from build123d import *

# Parameters (mm, degrees)
F0_R        = 4.945
F0_R_2      = 3.445
F1_DEPTH    = 4
F0_R_3      = 6.945
F1_FACE_R   = 4.945
F1_FACE_R_2 = 3.445
F2_DEPTH    = 1
F3_SIZE     = 0.99999
F4_SIZE2    = 1
F4_SIZE     = 1


# Not quite as in the source:
# - a fillet or chamfer is up to 0.001 mm smaller than in the source, because OpenCascade refuses the exact size


with BuildPart() as f1:
    # F0 (on Top) → F1 (new body)
    with BuildSketch(Plane.XY):
        Circle(F0_R)
        Circle(F0_R_2, mode=Mode.SUBTRACT)
    extrude(amount=-F1_DEPTH)

    # F0 (on Top) + F1_face (on face) → F2 (join)
    with BuildSketch(Plane.XY):
        Circle(F0_R_3)
        Circle(F0_R, mode=Mode.SUBTRACT)
        Circle(F0_R_2)
    with BuildSketch(Plane.XY):
        Circle(F1_FACE_R)
        Circle(F1_FACE_R_2, mode=Mode.SUBTRACT)
    extrude(amount=F2_DEPTH)

    # F3 (size 1 in the source; OpenCascade refuses exactly that, so slightly less here)
    f3_edges = [f1.edges().sort_by_distance(p)[0] for p in [
        (-6.945, 0, 1),
    ]]
    chamfer(f3_edges, length=F3_SIZE)

    # F4
    f4_edges = [f1.edges().sort_by_distance(p)[0] for p in [
        (-4.945, 0, -4),
    ]]
    chamfer(f4_edges, length=F4_SIZE, length2=F4_SIZE2)


solid = f1.part
Input: part model. Units: mm. Frame: model coordinates. A direction names the side the tool comes from. Coordinates: 2 decimals unless noted, no trailing zeros. Loops run counter-clockwise (first coordinate to the right, second up) from the corner with the lowest first, then second, coordinate; pieces in that order, holes last.
Q1. Set-up query: faces 4 (the face through (-2, 5, 0)), 5 (the face through (2, -3, -4)). Return all of +Z, -Z, +X, -X, +Y, -Y with unobstructed straight access to the full face (end or side cutting, diameter ignored); none if empty.
Q2. Cut plane D-D (z = 0.3). Output: boundary loops of the cut face in (x, y) (3 decimals).
Q3. Contact query for flat-ended pins moving along their axis: pin 1 (1.5 mm diameter, centred on y = 4, z = -2, fed in from +X); pin 2 (1 mm diameter, centred on x = -5, y = -3, fed in from -Z). Output: stop coordinate, or through.
Q4. Cut plane B-B (z = -1.1). Output: boundary loops of the cut face in (x, y) (3 decimals), then the cut area to 3 significant figures.
Q5. Material intervals for line 1 (Y direction, x = 0, z = -1.6) (3 decimals); line 2 (Z direction, x = 5, y = 3); line 3 (X direction, y = 2.75, z = -2.25), sorted ascending.
Q6. Draft query along Y for faces 1 (the face through (2.66, 4.17, -1.48)), 2 (the face through (0, 0, 0)), 3 (the face through (0, 0, 1)). Return one class per face: +Y half, -Y half, draft (parallel to the pull), parting line (faces both ways), or undercut.
Working result:
1. face 4: -Z
1. face 5: -Z, +X, -X, +Y, -Y
2. outline: circle Ø13.29 at (0, 0)
3. pin 1: stops at x = 3.73
3. pin 2: stops at z = 0
4. outline: circle Ø9.89 at (0, 0); hole circle Ø6.89 at (0, 0)
4. area: 39.5 mm2
5. line 1: y = -4.945 to -3.445, 3.445 to 4.945
5. line 2: z = 0 to 1
5. line 3: x = -4.11 to -2.07, 2.07 to 4.11
6. face 1: parting line
6. face 2: undercut
6. face 3: draft
